```python
from build123d import *

# Parameters (mm, degrees)
PAD_DEPTH       = 15
POCKET_DEPTH    = 4
POCKET001_DEPTH = 4
PAD001_DEPTH    = 2
POCKET002_DEPTH = 4
POCKET003_DEPTH = 4
SKETCH006_W     = 1.060891
SKETCH006_H     = 4.93171
POCKET004_DEPTH = 4
SKETCH007_W     = 1.038232
SKETCH007_H     = 4.977957
POCKET005_DEPTH = 4


with BuildPart() as part:
    # Sketch → Pad (new body)
    with BuildSketch(Plane.XY):
        Polygon((-10.147716, -10.055362), (9.967627, -10.055362), (9.967627, 0), (20.083433, 9.943707), (9.967627, 24.129093), (-9.915169, 24.129093), (-20.030979, 9.711162), (-10.147716, 0), align=None)
    extrude(amount=PAD_DEPTH)

    # Sketch001 (on Face10 of Pad) → Pocket (cut)
    with BuildSketch(Plane.XY.offset(15)):
        Polygon((-8.015594, 12.653538), (-6.378841, 17.407913), (-4.586209, 12.653538), align=None)
    extrude(amount=-POCKET_DEPTH, mode=Mode.SUBTRACT)

    # Sketch002 (on Face5 of Pocket) → Pocket001 (cut)
    with BuildSketch(Plane.XY.offset(15)):
        Polygon((3.209776, 12.792396), (4.256241, 17.210794), (6.232895, 12.908666), align=None)
    extrude(amount=-POCKET001_DEPTH, mode=Mode.SUBTRACT)

    # Sketch003 (on Face5 of Pocket001) → Pad001 (join)
    with BuildSketch(Plane.XY.offset(15)):
        Polygon((-0.640232, 8.644424), (-2.363165, 4.113749), (3.507571, 4.113749), align=None)
    extrude(amount=PAD001_DEPTH)

    # Sketch004 (on Face5 of Pad001) → Pocket002 (cut)
    with BuildSketch(Plane.XY.offset(15)):
        Polygon((-4.047933, -2.089132), (-4.047933, -7.000175), (-2.950786, -7.000175), (-2.950786, -2.036887), align=None)
    extrude(amount=-POCKET002_DEPTH, mode=Mode.SUBTRACT)

    # Sketch005 (on Face5 of Pocket002) → Pocket003 (cut)
    with BuildSketch(Plane.XY.offset(15)):
        Polygon((-2.046365, -1.977987), (-2.046365, -6.985984), (-0.855654, -7.056026), (-1.030757, -2.08305), align=None)
    extrude(amount=-POCKET003_DEPTH, mode=Mode.SUBTRACT)

    # Sketch006 (on Face5 of Pocket003) → Pocket004 (cut)
    with BuildSketch(Plane.XY.offset(15)):
        with Locations((0.70562, -4.49912)):
            Rectangle(SKETCH006_W, SKETCH006_H)
    extrude(amount=-POCKET004_DEPTH, mode=Mode.SUBTRACT)

    # Sketch007 (on Face5 of Pocket004) → Pocket005 (cut)
    with BuildSketch(Plane.XY.offset(15)):
        with Locations((2.627853, -4.495738)):
            Rectangle(SKETCH007_W, SKETCH007_H)
    extrude(amount=-POCKET005_DEPTH, mode=Mode.SUBTRACT)


solid = part.part
```
For this review, take the finished solid that the model builds, in its own axes (mm). A direction names the side the tool comes from. Coordinates: 2 decimals unless noted, no trailing zeros. Write each loop counter-clockwise with the first axis right and the second up, starting at its lowest first coordinate (ties: lowest second). Pieces come first, ordered by that corner, then holes. Notation, with made-up numbers: (-26.75, -1.75) - (11.25, -1.75) arc R23 ccw to (11.25, 28.25) - close; hole circle Ø9 at (-20, 77). An arc over 180 degrees is marked (long way). Answer in a Markdown table with one row per item. Add a question column.
Q1. For P1, Ø3, axis at y = -5.5, z = 12.5, coming from the -X side; P2, Ø3, axis at y = -4.5, z = 13.5, coming from the +X side; P3, Ø1.1, axis at x = 2.5, y = -4, coming from the +Z side, all flat-tipped, find the tip position at first contact; note any pin that passes through.
Q2. We need section C-C, the plane x = 7.5. State the section outline as (y, z) points, and give its area (3 significant figures).
Q3. We need section A-A, the plane z = 3.25. State the section outline as (x, y) points, and give its area (3 significant figures).
Q4. Draft analysis for pull direction X (two halves, no side actions). For faces 3 (the flat face through (0, 11, 15)), 4 (the flat face through (1.46, 6.35, 15.99)), 5 (the flat face through (5, 14, 11)), 6 (the flat face through (-15.159, 4.924, 7.395)), state which applies: +X half, -X half, draft (parallel to the pull), parting line (faces both ways), or undercut.
Q5. For probe 1 along X at (y, z) = (13.5, 13.75); probe 2 along Y at (x, z) = (-2, 11.75); probe 3 along Z at (x, y) = (-3, 14), list the stretches that pass through material, from the lowest coordinate up.
Q6. We need section D-D, the plane y = 6. State the section outline as (x, z) points, and give its area (3 significant figures).
Q7. We need section B-B, the plane y = 14. State the section outline as (x, z) points.
Q8. Tool access review of faces 1 (the flat face through (-14.902, 17.021, 7.395)), 2 (the flat face through (-2.046, -4, 13)): name each direction out of +Z, -Z, +X, -X, +Y, -Y from which nothing blocks a thin tool from reaching the whole face with its end or side.
Answer list:
| question | item | result |
|---|---|---|
| 1 | P1 | stops at x = -10.15 |
| 1 | P2 | stops at x = 9.97 |
| 1 | P3 | stops at z = 15 |
| 2 | outline | (-10.06, 0) - (24.13, 0) - (24.13, 15) - (-10.06, 15) - close |
| 2 | area | 513 mm2 |
| 3 | outline | (-20.03, 9.71) - (-10.15, 0) - (-10.15, -10.06) - (9.97, -10.06) - (9.97, 0) - (20.08, 9.94) - (9.97, 24.13) - (-9.92, 24.13) - close |
| 3 | area | 927 mm2 |
| 4 | face 3 | draft |
| 4 | face 4 | +X half |
| 4 | face 5 | undercut |
| 4 | face 6 | -X half |
| 5 | probe 1 | x = -17.37 to -7.72, -4.91 to 3.38, 5.96 to 17.55 |
| 5 | probe 2 | y = -10.06 to -6.99, -1.98 to 24.13 |
| 5 | probe 3 | z = 0 to 15 |
| 6 | outline | (-16.25, 0) - (16.07, 0) - (16.07, 15) - (1.78, 15) - (1.78, 17) - (-1.65, 17) - (-1.65, 15) - (-16.25, 15) - close |
| 6 | area | 492 mm2 |
| 7 | outline | (-17.02, 0) - (17.19, 0) - (17.19, 15) - (5.73, 15) - (5.73, 11) - (3.5, 11) - (3.5, 15) - (-5.09, 15) - (-5.09, 11) - (-7.55, 11) - (-7.55, 15) - (-17.02, 15) - close |
| 8 | face 1 | +Z, -Z, -X, +Y |
| 8 | face 2 | +Z |
